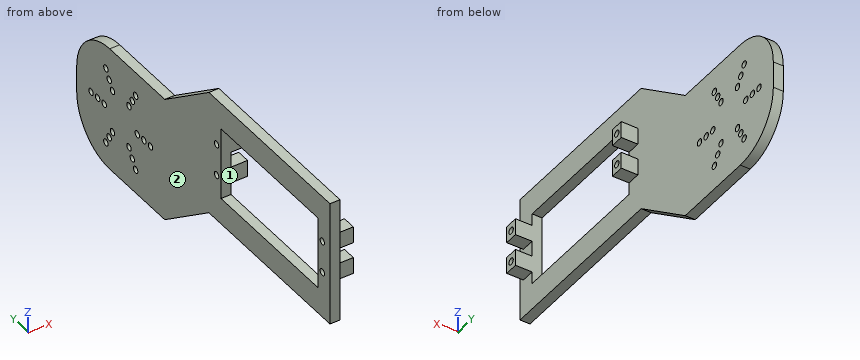
from build123d import *

# Parameters (mm, degrees)
SKETCH1_R           = 1
SKETCH1_W           = 22
SKETCH1_H           = 44
BOSS_EXTRUDE1_DEPTH = 1.5
FILLET1_R           = 15
SKETCH2_W           = 5
SKETCH2_H           = 4
SKETCH2_R           = 1
BOSS_EXTRUDE2_DEPTH = 5


with BuildPart() as part:
    # Sketch1 → Boss-Extrude1 (new, symmetric)
    with BuildSketch(Plane(origin=(0, 0, 0), x_dir=(0, 0, -1), z_dir=(1, 0, 0))):
        Polygon((-19, -27.5), (19, -27.5), (19, 27.5), (34, 47.5), (34, 87.5), (-4, 87.5), (-4, 47.5), (-19, 27.5), align=None)
        with Locations((-4.85, -24)):
            Circle(SKETCH1_R, mode=Mode.SUBTRACT)
        with Locations((4.85, -24)):
            Circle(SKETCH1_R, mode=Mode.SUBTRACT)
        with Locations((4.85, 24)):
            Circle(SKETCH1_R, mode=Mode.SUBTRACT)
        with Locations((-4.85, 24)):
            Circle(SKETCH1_R, mode=Mode.SUBTRACT)
        with Locations((15, 75)):
            Circle(SKETCH1_R, mode=Mode.SUBTRACT)
        with Locations((15, 78)):
            Circle(SKETCH1_R, mode=Mode.SUBTRACT)
        with Locations((15, 81)):
            Circle(SKETCH1_R, mode=Mode.SUBTRACT)
        with Locations((21.495190528, 71.25)):
            Circle(SKETCH1_R, mode=Mode.SUBTRACT)
        with Locations((24.09326674, 72.75)):
            Circle(SKETCH1_R, mode=Mode.SUBTRACT)
        with Locations((26.691342951, 74.25)):
            Circle(SKETCH1_R, mode=Mode.SUBTRACT)
        with Locations((21.495190528, 63.75)):
            Circle(SKETCH1_R, mode=Mode.SUBTRACT)
        with Locations((24.09326674, 62.25)):
            Circle(SKETCH1_R, mode=Mode.SUBTRACT)
        with Locations((26.691342951, 60.75)):
            Circle(SKETCH1_R, mode=Mode.SUBTRACT)
        with Locations((15, 60)):
            Circle(SKETCH1_R, mode=Mode.SUBTRACT)
        with Locations((15, 57)):
            Circle(SKETCH1_R, mode=Mode.SUBTRACT)
        with Locations((15, 54)):
            Circle(SKETCH1_R, mode=Mode.SUBTRACT)
        with Locations((8.504809472, 63.75)):
            Circle(SKETCH1_R, mode=Mode.SUBTRACT)
        with Locations((5.90673326, 62.25)):
            Circle(SKETCH1_R, mode=Mode.SUBTRACT)
        with Locations((3.308657049, 60.75)):
            Circle(SKETCH1_R, mode=Mode.SUBTRACT)
        with Locations((8.504809472, 71.25)):
            Circle(SKETCH1_R, mode=Mode.SUBTRACT)
        with Locations((5.90673326, 72.75)):
            Circle(SKETCH1_R, mode=Mode.SUBTRACT)
        with Locations((3.308657049, 74.25)):
            Circle(SKETCH1_R, mode=Mode.SUBTRACT)
        Rectangle(SKETCH1_W, SKETCH1_H, mode=Mode.SUBTRACT)
    extrude(amount=BOSS_EXTRUDE1_DEPTH, both=True)

    # Fillet1
    fillet1_edges = [part.edges().sort_by_distance(p)[0] for p in [
        (0, 87.5, 4),
        (0, 87.5, -34),
    ]]
    fillet(fillet1_edges, radius=FILLET1_R)

    # Sketch2 → Boss-Extrude2 (add)
    # profile 1 of 4: a face of its own
    with BuildSketch(Plane(origin=(1.5, 0, 0), x_dir=(0, 0, -1), z_dir=(1, 0, 0))):
        with Locations((-4.85, -24)):
            Rectangle(SKETCH2_W, SKETCH2_H)
        with Locations((-4.85, -24)):
            Circle(SKETCH2_R, mode=Mode.SUBTRACT)
    # profile 2 of 4: a face of its own
    with BuildSketch(Plane(origin=(1.5, 0, 0), x_dir=(0, 0, -1), z_dir=(1, 0, 0))):
        with Locations((4.85, -24)):
            Rectangle(SKETCH2_W, SKETCH2_H)
        with Locations((4.85, -24)):
            Circle(SKETCH2_R, mode=Mode.SUBTRACT)
    # profile 3 of 4: a face of its own
    with BuildSketch(Plane(origin=(1.5, 0, 0), x_dir=(0, 0, -1), z_dir=(1, 0, 0))):
        with Locations((4.85, 24)):
            Rectangle(SKETCH2_W, SKETCH2_H)
        with Locations((4.85, 24)):
            Circle(SKETCH2_R, mode=Mode.SUBTRACT)
    # profile 4 of 4: a face of its own
    with BuildSketch(Plane(origin=(1.5, 0, 0), x_dir=(0, 0, -1), z_dir=(1, 0, 0))):
        with Locations((-4.85, 24)):
            Rectangle(SKETCH2_W, SKETCH2_H)
        with Locations((-4.85, 24)):
            Circle(SKETCH2_R, mode=Mode.SUBTRACT)
    extrude(amount=BOSS_EXTRUDE2_DEPTH)


solid = part.part
For this review, take the finished solid that the model builds, in its own axes (mm). Face numbers are marked on the shaded views. Give positions to 0.01 mm unless a question says otherwise; leave off trailing zeros. Order: outer loops, then holes, each group sorted by start corner. A loop starts at its lowest first (then second) coordinate and runs counter-clockwise, first axis right, second up. Notation, with made-up numbers: M -11,-33 L 10,-33 A18 ccw 10,-20 Z; hole C 67.25,69.25 d5. An arc over 180 degrees is marked long. Answer in a Markdown table with one row per item. Add a question column.
(1) Consider section C-C on y = 67. State the section outline as (x, z) points.
(2) Mouldability with a two-part tool opening along Y and no side actions: class the marked faces 1 and 2 as +Y half, -Y half, draft (parallel to the pull), parting line (faces both ways), or undercut.
(3) Consider section A-A on x = 5.25. State the section outline as (y, z) points.
(4) For pin 1 (1.6 mm diameter, centred on y = 60.75, z = -3.31, fed in from +X); pin 2 (4 mm diameter, centred on x = 4.5, z = 6, fed in from +Y); pin 3 (2.5 mm diameter, centred on y = 54, z = -15, fed in from +X); pin 4 (4.5 mm diameter, centred on x = 3, y = -24.5, fed in from -Z), all flat-tipped, find the tip position at first contact; note any pin that passes through.
(5) Consider section D-D on z = 15. State the section outline as (x, y) points.
(6) Consider section B-B on y = -2.5. State the section outline as (x, z) points, and give its area (3 significant figures).
(7) Wall thickness on probe 1 along Y at (x, z) = (2.5, 3.5); probe 2 along Z at (x, y) = (-0.75, -2.5); probe 3 along Y at (x, z) = (-0.75, -4.5): over which ranges is each line inside the solid? List them lowest first. Write a range as [from, to].
Evaluation:
| question | item | result |
|---|---|---|
| 1 | outline | M -1.5,-34 L 1.5,-34 L 1.5,4 L -1.5,4 Z |
| 2 | face 1 | undercut |
| 2 | face 2 | draft |
| 3 | outline | M -26,-7.35 L -22,-7.35 L -22,-2.35 L -26,-2.35 Z; M -26,2.35 L -22,2.35 L -22,7.35 L -26,7.35 Z; M 22,-7.35 L 26,-7.35 L 26,-2.35 L 22,-2.35 Z; M 22,2.35 L 26,2.35 L 26,7.35 L 22,7.35 Z; hole C -24,-4.85 d2; hole C -24,4.85 d2; hole C 24,-4.85 d2; hole C 24,4.85 d2 |
| 4 | pin 1 | passes through |
| 4 | pin 2 | stops at y = 26 |
| 4 | pin 3 | stops at x = 1.5 |
| 4 | pin 4 | stops at z = -19 |
| 5 | outline | M -1.5,-27.5 L 1.5,-27.5 L 1.5,32.83 L -1.5,32.83 Z |
| 6 | outline | M -1.5,-19 L 1.5,-19 L 1.5,-11 L -1.5,-11 Z; M -1.5,11 L 1.5,11 L 1.5,19 L -1.5,19 Z |
| 6 | area | 48.0 mm^2 |
| 7 | probe 1 | y = [-26, -22], [22, 26] |
| 7 | probe 2 | z = [-19, -11], [11, 19] |
| 7 | probe 3 | y = [-27.5, -24.94], [-23.06, -22], [22, 23.06], [24.94, 86.02] |
